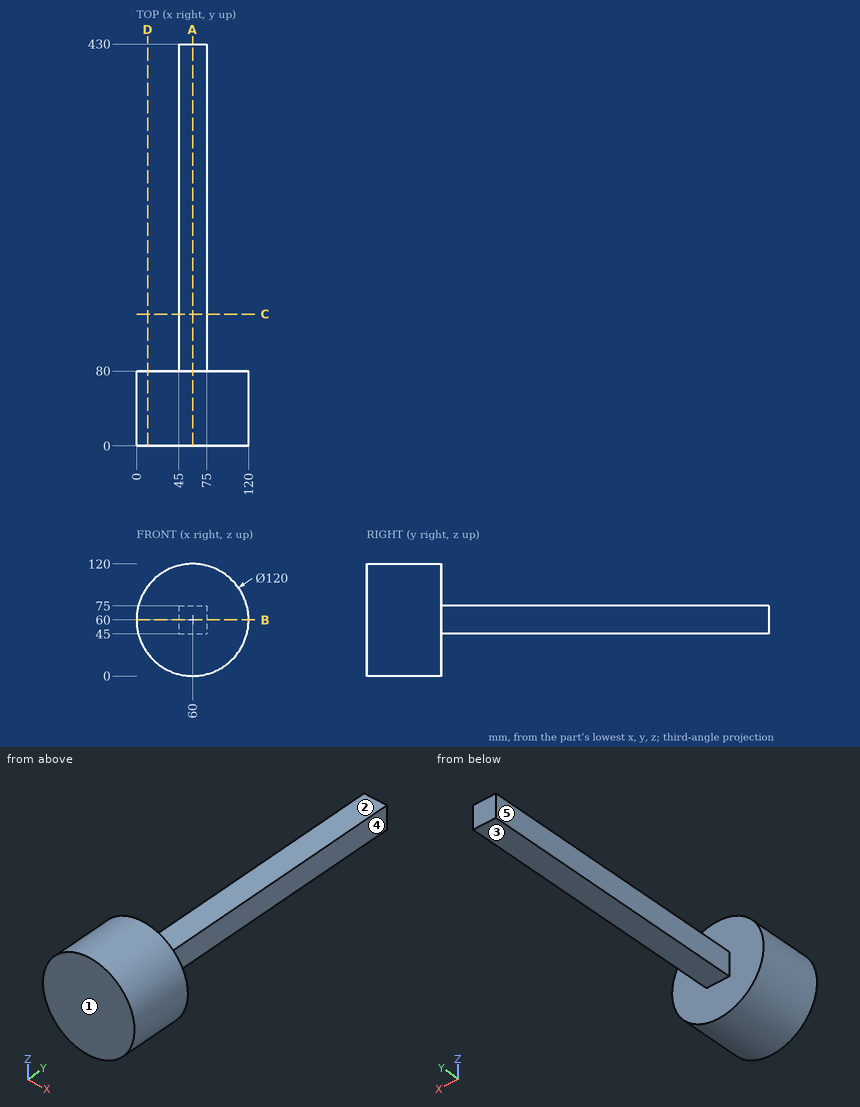
For this review, use the dimensioned drawing (mm, ordinates from the lowest corner) and the shaded views. A direction names the side the tool comes from. Coordinates: 2 decimals unless noted, no trailing zeros. Order: outer loops, then holes, each group sorted by start corner. A loop starts at its lowest first (then second) coordinate and runs counter-clockwise, first axis right, second up. Notation, with made-up numbers: (40.5, 12) -> (47.5, 12) arc R24 cw to (47.5, 43) -> close; hole circle Ø3 at (66.5, 40). An arc over 180 degrees is marked (long way). One line per item, written item: value. Start each with the question number.
Q1. Take a section at C-C, the plane y = 141. State the section outline as (x, z) points, then the cut area to 3 significant figures.
Q2. Take a section at D-D, the plane x = 12. State the section outline as (y, z) points.
Q3. Tool access review of the marked faces 1, 2, 3, 4 and 5: name each direction out of +Z, -Z, +X, -X, +Y, -Y from which nothing blocks a thin tool from reaching the whole face with its end or side.
Q4. Take a section at B-B, the plane z = 60. State the section outline as (x, y) points, then the cut area to 3 significant figures.
Q5. Insertion check: pin 1 Ø1 at (x, z) = (18, 24.5) entering from +Y; pin 2 Ø15 at (y, z) = (296, 58) entering from +X; pin 3 Ø15 at (x, y) = (65.5, 188) entering from -Z. Each pin has a flat end and moves straight along its axis. Give the tip position at first contact, or say it passes through.
Q6. For probe 1 along Z at (x, y) = (73.5, 115); probe 2 along Y at (x, z) = (25.5, 100.5); probe 3 along X at (y, z) = (47, 35), list the stretches that pass through material, from the lowest coordinate up.
Q7. Take a section at A-A, the plane x = 60. State the section outline as (y, z) points, then the cut area to 3 significant figures.
Values follow:
1. outline: (45, 45) -> (75, 45) -> (75, 75) -> (45, 75) -> close
1. area: 900 mm2
2. outline: (0, 24) -> (80, 24) -> (80, 96) -> (0, 96) -> close
3. face 1: +Z, -Z, +X, -X, -Y
3. face 2: +Z, +X, -X, +Y
3. face 3: -Z, +X, -X, +Y
3. face 4: +Z, -Z, +X, +Y
3. face 5: +Z, -Z, -X, +Y
4. outline: (0, 0) -> (120, 0) -> (120, 80) -> (75, 80) -> (75, 430) -> (45, 430) -> (45, 80) -> (0, 80) -> close
4. area: 20,100 mm2
5. pin 1: stops at y = 80
5. pin 2: stops at x = 75
5. pin 3: stops at z = 45
6. probe 1: z = 45 to 75
6. probe 2: y = 0 to 80
6. probe 3: x = 5.46 to 114.54
7. outline: (0, 0) -> (80, 0) -> (80, 45) -> (430, 45) -> (430, 75) -> (80, 75) -> (80, 120) -> (0, 120) -> close
7. area: 20,100 mm2
